Solid Edge part; units mm, degrees
sketch "Sketch1" plane through (0, 0, 0) normal (0, -1, 0) x (1, 0, 0)
  line L0 (-117, 12.5) -> (-113.75, 12.5)
  line L1 (-113.75, 12.5) -> (-113.75, 17)
  line L2 (-113.75, 17) -> (-108.25, 17)
  line L3 (-108.25, 17) -> (-108.25, 12.5)
  line L4 (-108.25, 12.5) -> (-105, 12.5)
  line L5 (-105, 12.5) -> (-105, -12.5)
  line L6 (-105, -12.5) -> (-108.25, -12.5)
  line L7 (-108.25, -12.5) -> (-108.25, -17)
  line L8 (-108.25, -17) -> (-113.75, -17)
  line L9 (-113.75, -17) -> (-113.75, -12.5)
  line L10 (-113.75, -12.5) -> (-117, -12.5)
  line L11 (-117, -12.5) -> (-117, 12.5)
  dimension "D1" = 108.25
  dimension "D2" = 108.25
  dimension "D3" = 113.75
  dimension "D4" = 105
  dimension "D5" = 117
  dimension "D6" = 108.25
  dimension "D7" = 113.75
  dimension "D8" = 108.25
  dimension "D9" = 105
revolve "RevolvedProtrusion1" add sketch "Sketch1" angle 10 about axis through (0, 0, 54) along (0, 0, 1)
properties material "ABS Plastic, high impact"
Could you check a few things on this model? Use its own coordinates, in mm. A direction names the side the tool comes from. Round coordinates to 2 decimals unless told otherwise and drop trailing zeros. Write each loop counter-clockwise with the first axis right and the second up, starting at its lowest first coordinate (ties: lowest second). Pieces come first, ordered by that corner, then holes. Notation, with made-up numbers: (61.5, 15) -> (78.5, 15) arc R25 cw to (78.5, 39) -> close; hole circle Ø6 at (27.5, 30). An arc over 180 degrees is marked (long way). Use a Markdown table: item, result.
1. If we section it at D-D (z = -7.5): List the corners of the cut face in (x, y) for me.
Answer key:
| item | result |
|---|---|
| outline | (-117, 0) arc R117 ccw to (-115.22, -20.32) -> (-103.4, -18.23) arc R105 cw to (-105, 0) -> close |
2. If we section it at C-C (y = -11.75): List the corners of the cut face in (x, z) for me, then the cut area to 3 significant figures.
Answer key:
| item | result |
|---|---|
| outline | (-116.41, -12.5) -> (-113.14, -12.5) -> (-113.14, -17) -> (-107.61, -17) -> (-107.61, -12.5) -> (-104.34, -12.5) -> (-104.34, 12.5) -> (-107.61, 12.5) -> (-107.61, 17) -> (-113.14, 17) -> (-113.14, 12.5) -> (-116.41, 12.5) -> close |
| area | 351 mm^2 |
3. For pin 1 Ø3 at (x, y) = (-115, -11) entering from +Z; pin 2 Ø12 at (y, z) = (-13, 2) entering from -X; pin 3 Ø1.5 at (y, z) = (-17.5, -11.5) entering from -X, each with a flat end and sliding along its axis, tell me the tip position at first contact or that it passes through.
Answer key:
| item | result |
|---|---|
| pin 1 | stops at z = 12.5 |
| pin 2 | stops at x = -116.79 |
| pin 3 | stops at x = -115.79 |
4. If we section it at A-A (y = -6.5): List the corners of the cut face in (x, z) for me.
Answer key:
| item | result |
|---|---|
| outline | (-116.82, -12.5) -> (-113.56, -12.5) -> (-113.56, -17) -> (-108.05, -17) -> (-108.05, -12.5) -> (-104.8, -12.5) -> (-104.8, 12.5) -> (-108.05, 12.5) -> (-108.05, 17) -> (-113.56, 17) -> (-113.56, 12.5) -> (-116.82, 12.5) -> close |
5. Which directions (+Z, -Z, +X, -X, +Y, -Y) give clear straight access to the entire face, cutting with the end or side of a thin tool? Please do faces 1 (the face through (-114, -10, 12.5)), 2 (the face through (-114, -10, -12.5)), 3 (the face through (-106, -10, -12.5)).
Answer key:
| item | result |
|---|---|
| face 1 | +Z, -X, -Y |
| face 2 | -Z, -X, -Y |
| face 3 | -Z, +X, +Y |
6. Please list where these lines run through material, in increasing order: probe 1 along Z at (x, y) = (-104.5, -14.75); probe 2 along X at (y, z) = (-13.25, 10); probe 3 along Y at (x, z) = (-108, -2).
Answer key:
| item | result |
|---|---|
| probe 1 | z = -12.5 to 12.5 |
| probe 2 | x = -116.25 to -104.16 |
| probe 3 | y = -19.04 to 0 |
7. If we section it at B-B (z = 15): List the corners of the cut face in (x, y) for me.
Answer key:
| item | result |
|---|---|
| outline | (-113.75, 0) arc R113.75 ccw to (-112.02, -19.75) -> (-106.61, -18.8) arc R108.25 cw to (-108.25, 0) -> close |
